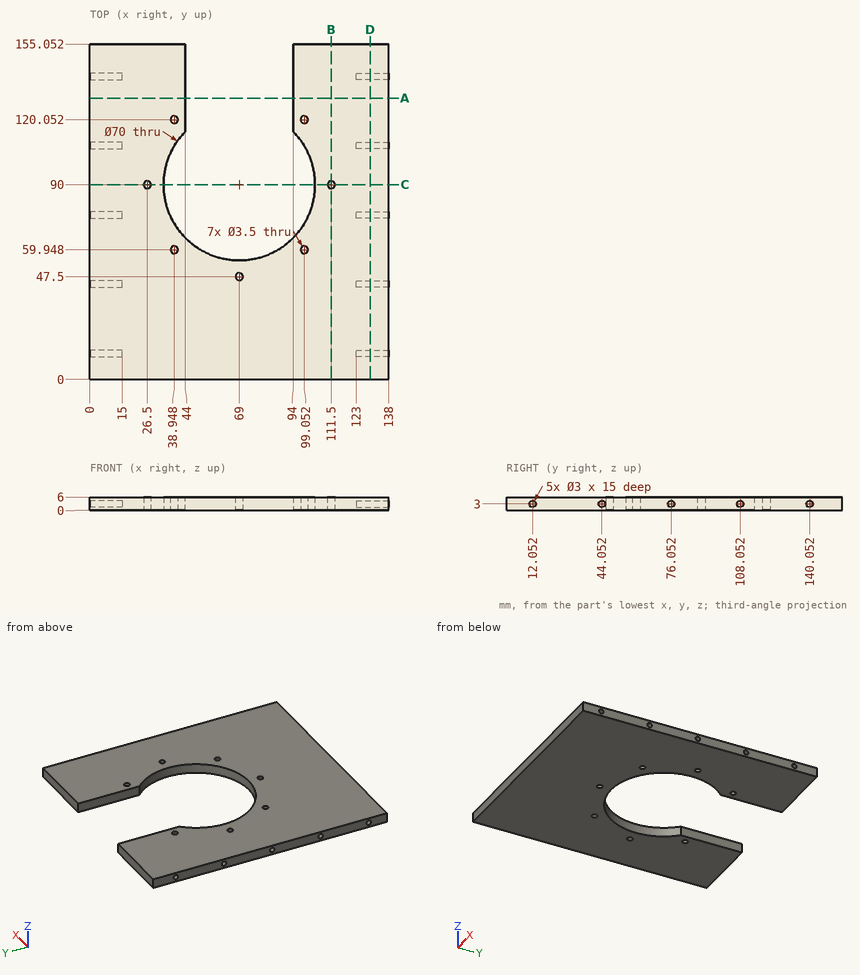
Geometry check sheet. Reference: drawing and pictorial views, mm from the part's lowest x, y, z. Round coordinates to 2 decimals unless told otherwise and drop trailing zeros. Order: outer loops, then holes, each group sorted by start corner. A loop starts at its lowest first (then second) coordinate and runs counter-clockwise, first axis right, second up. Notation, with made-up numbers: M 42.5,2 L 50.5,2 A14 cw 50.5,6 Z; hole C 42.5,36.25 d8. An arc over 180 degrees is marked long. One line per item, written item: value. Start each with the question number.
1. Section check B-B on x = 111.5. Enter the section's corners in (y, z), and give its area (3 significant figures).
2. Section check D-D on x = 129.5. Enter the section's corners in (y, z), and give its area (3 significant figures).
3. Section check C-C on y = 90. Enter the section's corners in (x, z).
4. Scan lines: line 1 along X through (y, z) = (91, 4.2); line 2 along X through (y, z) = (127.5, 4.65); line 3 along X through (y, z) = (90.5, 4.35). Record each from-to range of solid material in increasing order.
5. Section check A-A on y = 130. Enter the section's corners in (x, z).
6. Gauge pin test, flat ends, axial feed: P1, Ø0.9, axis at y = 11.5, z = 2.5, coming from the +X side; P2, Ø2.5, axis at y = 12.05, z = 3, coming from the -X side; P3, Ø2, axis at x = 76, z = 1, coming from the +Y side. Record the tip position at first contact, or that the pin passes through.
Results found:
1. outline: M 0,0 L 88.25,0 L 88.25,6 L 0,6 Z; M 91.75,0 L 155.05,0 L 155.05,6 L 91.75,6 Z
1. area: 909 mm^2
2. outline: M 0,0 L 155.05,0 L 155.05,6 L 0,6 Z; hole C 12.05,3 d3; hole C 44.05,3 d3; hole C 76.05,3 d3; hole C 108.05,3 d3; hole C 140.05,3 d3
2. area: 895 mm^2
3. outline: M 0,0 L 24.75,0 L 24.75,6 L 0,6 Z; M 28.25,0 L 34,0 L 34,6 L 28.25,6 Z; M 104,0 L 109.75,0 L 109.75,6 L 104,6 Z; M 113.25,0 L 138,0 L 138,6 L 113.25,6 Z
4. line 1: 0 to 25.06, 27.94 to 34.01, 103.99 to 110.06, 112.94 to 138
4. line 2: 0 to 44, 94 to 138
4. line 3: 0 to 24.82, 28.18 to 34, 104 to 109.82, 113.18 to 138
5. outline: M 0,0 L 44,0 L 44,6 L 0,6 Z; M 94,0 L 138,0 L 138,6 L 94,6 Z
6. P1: x = 123
6. P2: x = 15
6. P3: y = 55.93
